Could you check a few things on this model? Use its own coordinates, in mm. Face numbers are marked on the shaded views. Round coordinates to 2 decimals unless told otherwise and drop trailing zeros. Write each loop counter-clockwise with the first axis right and the second up, starting at its lowest first coordinate (ties: lowest second). Pieces come first, ordered by that corner, then holes. Notation, with made-up numbers: (57, -39) - (62, -39) arc R17 ccw to (62, -35) - close; hole circle Ø9 at (-29.75, 30.25). An arc over 180 degrees is marked (long way). Write each question's results on one line, items separated by ' | '. Start each with the question number.
(1) Please list where these lines run through material, in increasing order: line 1 (Y direction, x = 0, z = 7.75); line 2 (Z direction, x = -5.5, y = -7); line 3 (X direction, y = -21, z = 9.25). Write a range as [from, to].
(2) Thinking about a two-plate mould opening in Y: for the marked faces 1, 2, 3 and 4, which applies, +Y half, -Y half, draft (parallel to the pull), parting line (faces both ways), or undercut?
(3) Imagine slicing it at A-A on z = 3.5. Write out the boundary of the cut face in (x, y).
(4) Imagine slicing it at B-B on x = 0. Write out the boundary of the cut face in (y, z).
(5) For P1, Ø2, axis at x = 9, z = 3.5, coming from the -Y side; P2, Ø1, axis at y = -15.5, z = 3, coming from the +X side; P3, Ø0.6, axis at y = -6.5, z = 1, coming from the -X side, each with a flat end and sliding along its axis, tell me the tip position at first contact or that it passes through.
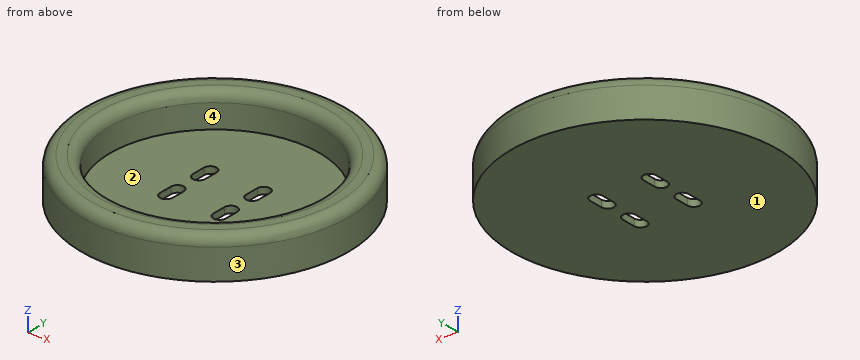
```python
from build123d import *

# Parameters (mm, degrees)
BOSS_EXTRUDE1_OUTLINE_R = 39.549034963
BOSS_EXTRUDE1_DEPTH     = 12
SKETCH2_R               = 30.977240476
CUT_EXTRUDE1_DEPTH      = 10
FILLET1_R               = 3
FILLET3_R               = 3
CUT_EXTRUDE2_DEPTH      = 10


# Read off the part's stored shape, not the designer's step: Boss-Extrude1
with BuildPart() as part:
    # Boss-Extrude1 outline → Boss-Extrude1 (new body)
    with BuildSketch(Plane.XY):
        Circle(BOSS_EXTRUDE1_OUTLINE_R)
    extrude(amount=BOSS_EXTRUDE1_DEPTH)

    # Sketch2 → Cut-Extrude1 (cut)
    with BuildSketch(Plane.XY.offset(12)):
        Circle(SKETCH2_R)
    extrude(amount=-CUT_EXTRUDE1_DEPTH, mode=Mode.SUBTRACT)

    # Fillet1
    fillet1_edges = [part.edges().sort_by_distance(p)[0] for p in [
        (-39.549034963, 0, 12),
    ]]
    fillet(fillet1_edges, radius=FILLET1_R)

    # Fillet3
    fillet3_edges = [part.edges().sort_by_distance(p)[0] for p in [
        (-30.977240476, 0, 12),
    ]]
    fillet(fillet3_edges, radius=FILLET3_R)

    # Sketch3 → Cut-Extrude2 (cut)
    with BuildSketch(Plane.XY.offset(2)):
        with BuildLine():
            Line((-6.044621496, 7.992332867), (-6.044621496, 3.895422742))
            ThreePointArc((-6.044621496, 3.895422742), (-7.925170406, 2.014873832), (-9.805719315, 3.895422742))
            Line((-9.805719315, 3.895422742), (-9.805719315, 7.992332867))
            ThreePointArc((-9.805719315, 7.992332867), (-7.925170406, 9.872881776), (-6.044621496, 7.992332867))
        make_face()
        with BuildLine():
            Line((6.044621496, 7.992332867), (6.044621496, 3.895422742))
            ThreePointArc((6.044621496, 3.895422742), (7.925170406, 2.014873832), (9.805719315, 3.895422742))
            Line((9.805719315, 3.895422742), (9.805719315, 7.992332867))
            ThreePointArc((9.805719315, 7.992332867), (7.925170406, 9.872881776), (6.044621496, 7.992332867))
        make_face()
        with BuildLine():
            Line((6.044621496, -7.992332867), (6.044621496, -3.895422742))
            ThreePointArc((6.044621496, -3.895422742), (7.925170406, -2.014873832), (9.805719315, -3.895422742))
            Line((9.805719315, -3.895422742), (9.805719315, -7.992332867))
            ThreePointArc((9.805719315, -7.992332867), (7.925170406, -9.872881776), (6.044621496, -7.992332867))
        make_face()
        with BuildLine():
            Line((-6.044621496, -7.992332867), (-6.044621496, -3.895422742))
            ThreePointArc((-6.044621496, -3.895422742), (-7.925170406, -2.014873832), (-9.805719315, -3.895422742))
            Line((-9.805719315, -3.895422742), (-9.805719315, -7.992332867))
            ThreePointArc((-9.805719315, -7.992332867), (-7.925170406, -9.872881776), (-6.044621496, -7.992332867))
        make_face()
    extrude(amount=-CUT_EXTRUDE2_DEPTH, mode=Mode.SUBTRACT)


solid = part.part
```
Response:
1) line 1: [-39.55, -30.98], [30.98, 39.55] | line 2: [0, 2] | line 3: [-33.5, -22.79], [22.79, 33.5]
2) face 1: draft | face 2: undercut | face 3: parting line | face 4: undercut
3) outline: circle Ø79.1 at (0, 0); hole circle Ø61.95 at (0, 0)
4) outline: (-39.55, 0) - (39.55, 0) - (39.55, 9) arc R3 ccw to (36.55, 12) - (33.98, 12) arc R3 ccw to (30.98, 9) - (30.98, 2) - (-30.98, 2) - (-30.98, 9) arc R3 ccw to (-33.98, 12) - (-36.55, 12) arc R3 ccw to (-39.55, 9) - close
5) P1: y = -38.73 | P2: x = 36.59 | P3: x = -39.06
